```python
from build123d import *

# Parameters (mm, degrees)
ESQUISSE1_R          = 2.5
BASE_EXTRUSION_DEPTH = 12.25


with BuildPart() as part:
    # Esquisse1 → Base-Extrusion (new body)
    with BuildSketch(Plane.XY):
        with BuildLine():
            Line((-6.5, 0), (-6.5, -49.575699692))
            ThreePointArc((-6.5, -49.575699692), (0, 50), (6.5, -49.575699692))
            Line((6.5, -49.575699692), (6.5, 0))
            ThreePointArc((6.5, 0), (0, 6.5), (-6.5, 0))
        make_face()
        with Locations((0, 40)):
            Circle(ESQUISSE1_R, mode=Mode.SUBTRACT)
    extrude(amount=BASE_EXTRUSION_DEPTH)


solid = part.part
```
Source: CAD feature listing. Evaluate the final solid. Frame: model axes, mm. A direction names the side the tool comes from. Give positions to 0.01 mm unless a question says otherwise; leave off trailing zeros. Write each loop counter-clockwise with the first axis right and the second up, starting at its lowest first coordinate (ties: lowest second). Pieces come first, ordered by that corner, then holes. Notation, with made-up numbers: (10, 49.5) - (17, 49.5) arc R19 ccw to (17, 82.5) - close; hole circle Ø11 at (16.25, 69.5). An arc over 180 degrees is marked (long way). One line per item, written item: value. Start each with the question number.
Q1. Section query B-B, the plane z = 10.75. Return the cut outline in (x, y), then the cut area to 3 significant figures.
Q2. Section query A-A, the plane y = 40. Return the cut outline in (x, z), then the cut area to 3 significant figures.
Q3. First-contact query: pin 1 Ø6 at (x, y) = (-1, -35) entering from -Z; pin 2 Ø1.5 at (y, z) = (-38.5, 7) entering from -X; pin 3 Ø2 at (x, z) = (-23, 5) entering from -Y; pin 4 Ø2 at (x, z) = (-29.5, 4.5) entering from -Y. Flat tips, straight axial feed; report the tip coordinate or a pass-through.
Q4. Section query D-D, the plane x = 4. Return the cut outline in (y, z), then the cut area to 3 significant figures.
Q5. Section query C-C, the plane y = -31. Return the cut outline in (x, z), then the cut area to 3 significant figures.
Q6. Set-up query: faces 4 (the face through (-6.5, -24, 6)), 5 (the face through (-2.107, 49.956, 6.039)). Return all of +Z, -Z, +X, -X, +Y, -Y with unobstructed straight access to the full face (end or side cutting, diameter ignored); none if empty.
Q7. Draft query along Y for faces 1 (the face through (0.1, 6.5, 6)), 2 (the face through (-10, 1, 0)), 3 (the face through (-0.54, 37.56, 6.04)). Return one class per face: +Y half, -Y half, draft (parallel to the pull), parting line (faces both ways), or undercut.
Q8. Material intervals for probe 1 along Y at (x, z) = (0, 6.5); probe 2 along X at (y, z) = (-22.5, 4.25); probe 3 along X at (y, z) = (5.5, 3.75), sorted ascending. Write a range as from..to.
Answer:
1. outline: (-6.5, -49.58) - (-6.5, 0) arc R6.5 cw to (6.5, 0) - (6.5, -49.58) arc R50 ccw (long way) to start; hole circle Ø5 at (0, 40)
1. area: 7,120 mm2
2. outline: (-30, 0) - (-2.5, 0) - (-2.5, 12.25) - (-30, 12.25) - close; (2.5, 0) - (30, 0) - (30, 12.25) - (2.5, 12.25) - close
2. area: 674 mm2
3. pin 1: passes through
3. pin 2: stops at x = -32.79
3. pin 3: stops at y = -44.9
3. pin 4: stops at y = -41.08
4. outline: (5.12, 0) - (49.84, 0) - (49.84, 12.25) - (5.12, 12.25) - close
4. area: 548 mm2
5. outline: (-39.23, 0) - (-6.5, 0) - (-6.5, 12.25) - (-39.23, 12.25) - close; (6.5, 0) - (39.23, 0) - (39.23, 12.25) - (6.5, 12.25) - close
5. area: 802 mm2
6. face 4: +Z, -Z, -Y
6. face 5: +Z, -Z
7. face 1: -Y half
7. face 2: draft
7. face 3: undercut
8. probe 1: y = 6.5..37.5, 42.5..50
8. probe 2: x = -44.65..-6.5, 6.5..44.65
8. probe 3: x = -49.7..-3.46, 3.46..49.7
